Check sheet for the modelled part. Datum: model origin and axes. Units: mm. A direction names the side the tool comes from. Round coordinates to 2 decimals unless told otherwise and drop trailing zeros. Write each loop counter-clockwise with the first axis right and the second up, starting at its lowest first coordinate (ties: lowest second). Pieces come first, ordered by that corner, then holes.
Item 1: Material ranges on line 1 (Z direction, x = 0, y = 7.75); line 2 (Y direction, x = -1.5, z = 9); line 3 (X direction, y = 2.75, z = 4), recorded low to high.
Item 2: Go/stop test with flat-tipped pins: pin 1 Ø5 at (y, z) = (3.5, 4.5) entering from -X; pin 2 Ø1.5 at (x, y) = (-5, 1) entering from +Z; pin 3 Ø8 at (x, z) = (0, 0) entering from +Y; pin 4 Ø6 at (x, y) = (-7.5, 8.5) entering from -Z. Record where each tip stops, or that it passes through.
Item 3: Cross-section at B-B on x = -4.25. Enter the section's corners in (y, z), plus the area to 3 significant figures.
Item 4: Tool access check on faces 1 (the flat face through (0, 2, 7)), 2 (the cylindrical face through (-2.17, 0.99, 9.76)). Record the directions out of +Z, -Z, +X, -X, +Y, -Y that give a thin tool (end or side, any length) a straight path to the whole face; none if there is none.
Item 5: Cross-section at D-D on z = 6.75. Enter the section's corners in (x, y).
Item 6: Release check for a two-part mould opening along X. For faces 3 (the cylindrical face through (-1.08, 4.93, -4.88)), 4 (the flat face through (-4, 10, 4)), 5 (the cylindrical face through (-6, 6, 0)) record: +X half, -X half, draft (parallel to the pull), parting line (faces both ways), or undercut.
Item 7: Cross-section at A-A on z = 0. Enter the section's corners in (x, y).
Item 8: Cross-section at C-C on y = 6. Enter the section's corners in (x, z), plus the area to 3 significant figures.
from build123d import *

# Parameters (mm, degrees)
SKETCH1_R           = 10
BOSS_EXTRUDE1_DEPTH = 2
SKETCH3_R           = 6
SKETCH3_R_2         = 5
BOSS_EXTRUDE2_DEPTH = 10
SKETCH4_R           = 5
CUT_EXTRUDE2_DEPTH  = 10


with BuildPart() as part:
    # Sketch1 → Boss-Extrude1 (new body)
    with BuildSketch(Plane(origin=(0, 0, 0), x_dir=(1, 0, 0), z_dir=(0, 1, 0))):
        Circle(SKETCH1_R)
    extrude(amount=BOSS_EXTRUDE1_DEPTH)

    # Sketch3 → Boss-Extrude2 (add)
    with BuildSketch(Plane.XZ):
        Circle(SKETCH3_R)
        Circle(SKETCH3_R_2, mode=Mode.SUBTRACT)
    extrude(amount=-BOSS_EXTRUDE2_DEPTH)

    # Sketch4 → Cut-Extrude2 (cut)
    with BuildSketch(Plane.XZ):
        Circle(SKETCH4_R)
    extrude(amount=-CUT_EXTRUDE2_DEPTH, mode=Mode.SUBTRACT)


solid = part.part
Response values:
1. line 1: z = -6 to -5, 5 to 6
1. line 2: y = 0 to 2
1. line 3: x = -4.47 to -3, 3 to 4.47
2. pin 1: stops at x = -9.68
2. pin 2: stops at z = 9.05
2. pin 3: passes through
2. pin 4: stops at z = -3.97
3. outline: (0, -9.05) - (2, -9.05) - (2, -4.24) - (10, -4.24) - (10, -2.63) - (0, -2.63) - close; (0, 2.63) - (10, 2.63) - (10, 4.24) - (2, 4.24) - (2, 9.05) - (0, 9.05) - close
3. area: 51.3 mm2
4. face 1: +Y
4. face 2: +Y, -Y
5. outline: (-7.38, 0) - (7.38, 0) - (7.38, 2) - (-7.38, 2) - close
6. face 3: undercut
6. face 4: draft
6. face 5: parting line
7. outline: (-10, 0) - (-5, 0) - (-5, 10) - (-6, 10) - (-6, 2) - (-10, 2) - close; (5, 0) - (10, 0) - (10, 2) - (6, 2) - (6, 10) - (5, 10) - close
8. outline: circle Ø12 at (0, 0); hole circle Ø10 at (0, 0)
8. area: 34.6 mm2
